```python
from build123d import *

# Parameters (mm, degrees)
F2_T = 2.5


# Not quite as in the source:
# - a shell that OpenCascade refuses in one call is made with other operations: the cavity is built on its own and cut out


with BuildPart() as f1:
    # F0 (on Front) → F1 (revolve)
    with BuildSketch(Plane.XZ):
        Polygon((0, 98.8223368999), (0, -101.1776631001), (43.9656563103, -101.1776631001), (43.9656563103, -97.5007638335), (5.4530212656, -90.7485485077), (5.4530212656, 55.7995252311), (50, 98.8223368999), align=None)
    revolve(axis=Axis((0, 0, -1.1776631001), (0, 0, 1)))

    # F2: shell of thickness 2.5, made by hand


with BuildPart() as f2_core1:
    # F2_t2: copy of F1
    add(f1.part)

    # the walls: a layer under each face that stays
    f2_faces = [f2_core1.faces().sort_by_distance(p)[0] for p in [
        (-27.7265106328, 0, 77.3109310655),
        (0, 0, -101.1776631001),
        (-43.9656563103, 0, -99.3392134668),
        (-24.7093387879, 0, -94.1246561706),
        (-5.4530212656, 0, -17.4745116383),
    ]]
    thicken(f2_faces, amount=-F2_T, mode=Mode.SUBTRACT)

    # F2_s3 → F2_t4 (revolve, cut)
    with BuildSketch(Plane.XZ):
        Polygon((5.4953886218, 55.7815426024), (3.7162856398, 57.5977881058), (2.9530212656, 56.8606386882), (2.9530212656, 55.7995252311), align=None)
    revolve(axis=Axis((0, 0, 55.7995252311), (0, 0, 1)), mode=Mode.SUBTRACT)

    # F2_s5 → F2_t6 (revolve, cut)
    with BuildSketch(Plane.XZ):
        Polygon((5.4823385311, -90.7239241048), (5.0212947153, -93.2109887985), (2.9530212656, -92.8483694226), (2.9530212656, -90.7485485077), align=None)
    revolve(axis=Axis((0, 0, -90.7485485077), (0, 0, 1)), mode=Mode.SUBTRACT)


with BuildPart() as f1_1:
    add(f1.part)

    # what is left inside the walls is the cavity
    f2_cavity = [f2_core1.part.solids().sort_by_distance(p)[0] for p in [
        (-17.927255, 0, 71.357287),
    ]]
    add(f2_cavity, mode=Mode.SUBTRACT)


solid = f1_1.part
```
Here's how the part is built. I have some questions about the finished solid (model axes, mm). A direction names the side the tool comes from. Round coordinates to 2 decimals unless told otherwise and drop trailing zeros. Write each loop counter-clockwise with the first axis right and the second up, starting at its lowest first coordinate (ties: lowest second). Pieces come first, ordered by that corner, then holes.
Q1. If we section it at A-A on z = -6.5: Write out the boundary of the cut face in (x, y).
Q2. If we section it at B-B on x = -31: Give the number of separate pieces and of enclosed holes in the cut face, plus the area to 3 significant figures.
Q3. Which directions (+Z, -Z, +X, -X, +Y, -Y) give clear straight access to the entire face, cutting with the end or side of a thin tool? Please do faces 4 (the flat face through (1, 1, -101.178)), 5 (the cylindrical face through (23.64, 37.07, -99.31)), 6 (the cylindrical face through (-1.182, -5.323, -16.449)).
Q4. Will these pins go through, and if not, where does the flat tip stop? P1, Ø12, axis at x = 17, y = -24.5, coming from the +Z side; P2, Ø21.5, axis at x = -15.5, y = 7.5, coming from the +Z side; P3, Ø1.5, axis at x = 6.5, y = -37.5, coming from the +Z side.
Q5. Please list where these lines run through material, in increasing order: probe 1 along Y at (x, z) = (0, -57); probe 2 along Z at (x, y) = (-6, 6); probe 3 along Z at (x, y) = (-11, -7).
Q6. If we mould it in two halves opening along Y, with no side actions, what happens to faces 1 (the conical face through (-0.953, 7.261, -91.076)), 2 (the flat face through (44.21, -14.58, 98.822)), 3 (the cylindrical face through (-2.95, 0.13, -16.95))? For each: +Y half, -Y half, draft (parallel to the pull), parting line (faces both ways), or undercut.
Answer below:
1. outline: circle Ø10.91 at (0, 0); hole circle Ø5.91 at (0, 0)
2. separate pieces: 2
2. enclosed holes: 1
2. area: 555 mm2
3. face 4: -Z, +X, -X, +Y, -Y
3. face 5: -Z
3. face 6: none
4. P1: stops at z = 88.6
4. P2: stops at z = 81.02
4. P3: stops at z = 91.49
5. probe 1: y = -5.45 to -2.95, 2.95 to 5.45
5. probe 2: z = -101.18 to -98.68, -93.82 to -91.28, 58.73 to 62.2
5. probe 3: z = -101.18 to -98.68, -94.62 to -92.08, 63.13 to 66.6
6. face 1: parting line
6. face 2: draft
6. face 3: undercut
